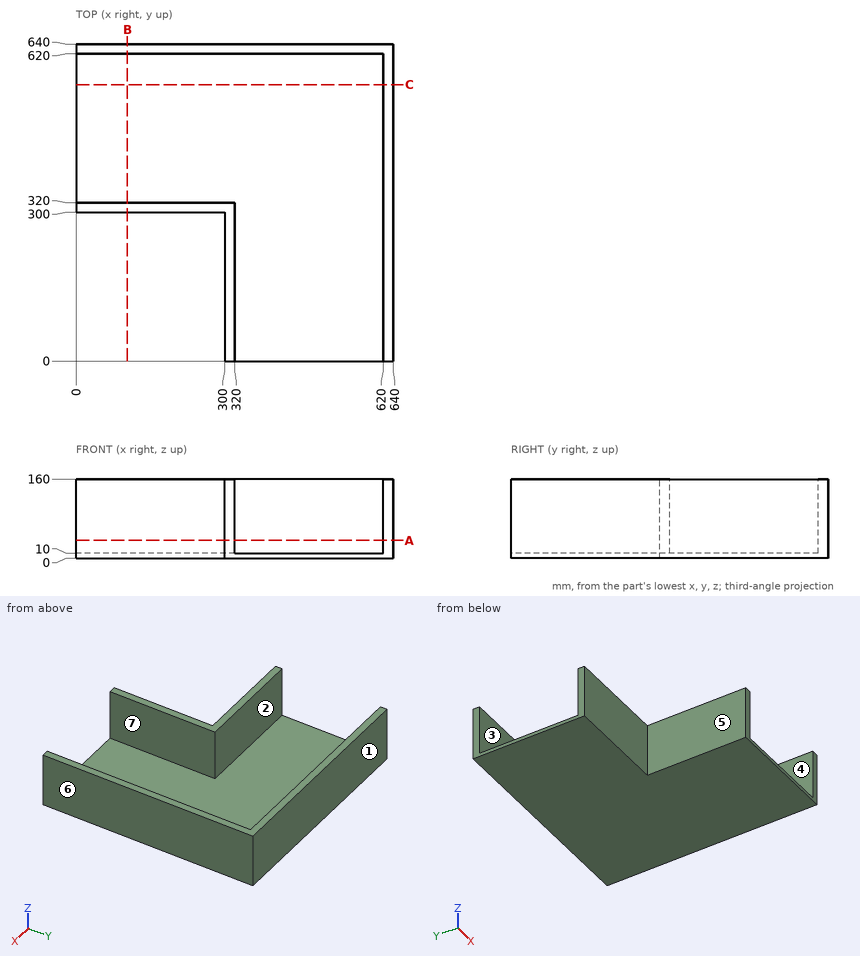
Source: three-view drawing plus pictorial views. Frame: mm from the lowest corner of the part. A direction names the side the tool comes from. Give positions to 0.01 mm unless a question says otherwise; leave off trailing zeros. Loops run counter-clockwise (first coordinate to the right, second up) from the corner with the lowest first, then second, coordinate; pieces in that order, holes last. Notation, with made-up numbers: (-36, 26) -> (15, 26) arc R30 cw to (15, 52) -> close; hole circle Ø9 at (-31.75, 20.25). An arc over 180 degrees is marked (long way). Put each result on its own line as item: value. Start each with the question number.
1) Cut plane A-A (z = 36). Return loops of the section in (x, y).
2) Material intervals for probe 1 along X at (y, z) = (168, 121); probe 2 along Y at (x, z) = (305.5, 101.5), sorted ascending.
3) Contact query for flat-ended pins moving along their axis: P1, Ø3, axis at x = 438, z = 105.5, coming from the -Y side; P2, Ø4, axis at y = 254.5, z = 57, coming from the -X side; P3, Ø1.5, axis at x = 162.5, z = 63, coming from the -Y side; P4, Ø12, axis at x = 303.5, y = 260.5, coming from the -Z side. Output: stop coordinate, or through.
4) Draft query along Y for the marked faces 1, 2, 3 and 4. Return one class per face: released by +Y, released by -Y, zero draft, split by the parting line, or undercut.
5) Reachability of the marked faces 5, 6 and 7 from +Z, -Z, +X, -X, +Y, -Y: full face, straight path, thin tool, end or side. Return the list, or none.
6) Cut plane B-B (x = 103.5). Return loops of the section in (y, z).
7) Cut plane C-C (y = 558). Return loops of the section in (x, z).
Results are:
1. outline: (0, 300) -> (300, 300) -> (300, 0) -> (320, 0) -> (320, 320) -> (0, 320) -> close; (0, 620) -> (620, 620) -> (620, 0) -> (640, 0) -> (640, 640) -> (0, 640) -> close
2. probe 1: x = 300 to 320, 620 to 640
2. probe 2: y = 0 to 320, 620 to 640
3. P1: stops at y = 620
3. P2: stops at x = 300
3. P3: stops at y = 300
3. P4: stops at z = 0
4. face 1: released by +Y
4. face 2: undercut
4. face 3: undercut
4. face 4: zero draft
5. face 5: +Z, -Z, -X, -Y
5. face 6: +Z, -Z, +X, +Y, -Y
5. face 7: +Z, -Y
6. outline: (300, 0) -> (640, 0) -> (640, 160) -> (620, 160) -> (620, 10) -> (320, 10) -> (320, 160) -> (300, 160) -> close
7. outline: (0, 0) -> (640, 0) -> (640, 160) -> (620, 160) -> (620, 10) -> (0, 10) -> close
